Geometry: see drawing. Coordinates: mm, zero at the bounding-box minimum. A direction names the side the tool comes from. Round coordinates to 2 decimals unless told otherwise and drop trailing zeros. Order: outer loops, then holes, each group sorted by start corner. A loop starts at its lowest first (then second) coordinate and runs counter-clockwise, first axis right, second up. Notation, with made-up numbers: (40, -0.5) -> (86, -0.5) arc R28 cw to (86, 32.5) -> close; hole circle Ø8 at (87.25, 86.25). An arc over 180 degrees is marked (long way). Answer as CSV lines item,"result". Start each with the question number.
(1) Section query A-A (x = 36). Output: boundary loops of the cut face in (y, z).
(2) Line query: line 1 along X through (y, z) = (3.8, 60.29); line 2 along X through (y, z) = (0.3, 5); line 3 along X through (y, z) = (3.5, 39.5). Output: solid intervals per line, ascending. Write a range as from..to.
(3) Contact query for flat-ended pins moving along their axis: P1, Ø0.9, axis at y = 1, z = 49.5, coming from the +X side; P2, Ø12, axis at x = 13.5, z = 42, coming from the -Y side; P3, Ø2.5, axis at y = 2, z = 37, coming from the -X side; P4, Ø1, axis at x = 16.5, z = 56.5, coming from the -Y side. Output: stop coordinate, or through.
(4) Section query C-C (y = 3.9). Output: boundary loops of the cut face in (x, z).
(5) Section query D-D (x = 23). Output: boundary loops of the cut face in (y, z), plus the area to 3 significant figures.
(6) Section query B-B (z = 5.5). Output: boundary loops of the cut face in (x, y).
(7) Set-up query: the marked faces 1, 2 and 3. Return all of +Z, -Z, +X, -X, +Y, -Y with unobstructed straight access to the full face (end or side cutting, diameter ignored); none if empty.
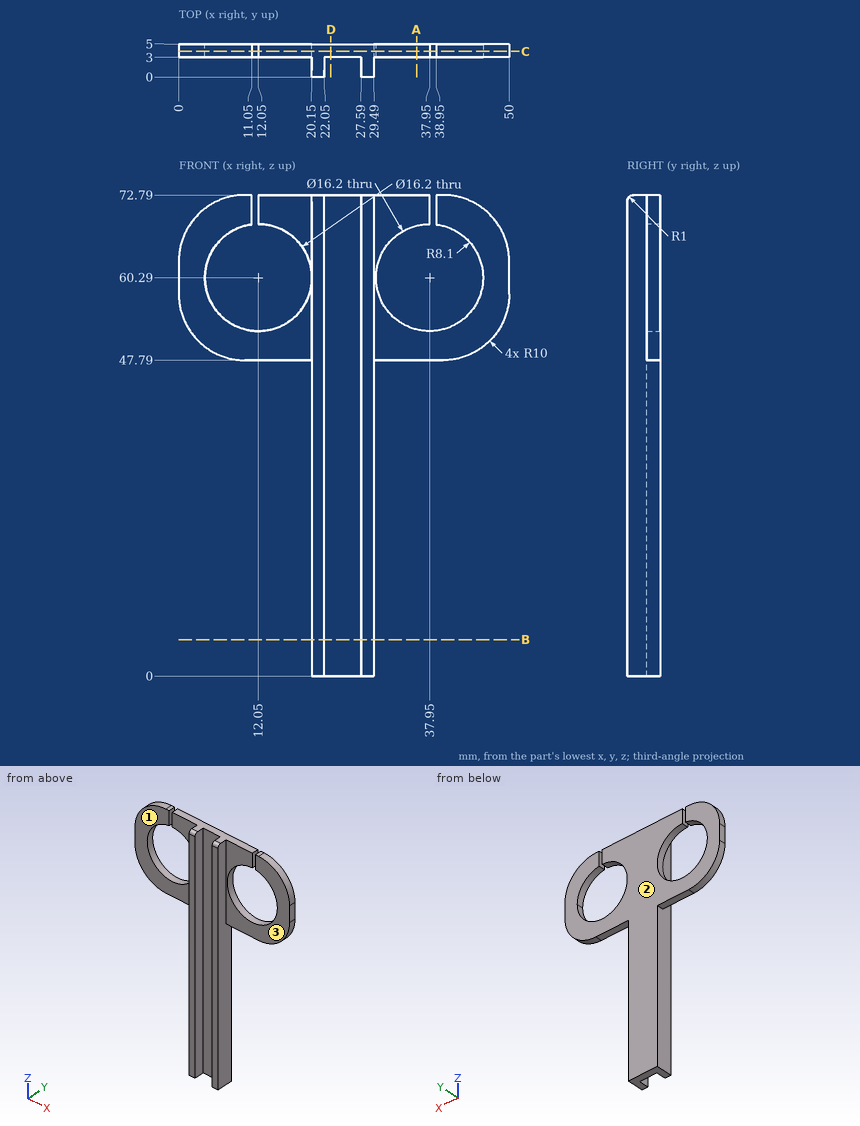
Answer block:
1,outline,"(3, 47.79) -> (5, 47.79) -> (5, 52.43) -> (3, 52.43) -> close; (3, 68.15) -> (5, 68.15) -> (5, 72.79) -> (3, 72.79) -> close"
2,line 1,"0..3.95, 20.15..29.85, 46.05..50"
2,line 2,"20.15..22.05, 27.59..29.49"
2,line 3,"20.15..29.49"
3,P1,"x = 29.49"
3,P2,"y = 3"
3,P3,"x = 20.15"
3,P4,"through"
4,outline,"(0, 57.79) arc R10 ccw to (10, 47.79) -> (20.15, 47.79) -> (20.15, 0) -> (29.49, 0) -> (29.49, 47.79) -> (40, 47.79) arc R10 ccw to (50, 57.79) -> (50, 62.79) arc R10 ccw to (40, 72.79) -> (38.95, 72.79) -> (38.95, 68.33) arc R8.1 cw (long way) to (37.95, 68.39) -> (37.95, 72.79) -> (12.05, 72.79) -> (12.05, 68.39) arc R8.1 cw (long way) to (11.05, 68.33) -> (11.05, 72.79) -> (10, 72.79) arc R10 ccw to (0, 62.79) -> close"
5,outline,"(3, 0) -> (5, 0) -> (5, 72.79) -> (3, 72.79) -> close"
5,area,"146 mm2"
6,outline,"(20.15, 0) -> (22.05, 0) -> (22.05, 3) -> (27.59, 3) -> (27.59, 0) -> (29.49, 0) -> (29.49, 5) -> (20.15, 5) -> close"
7,face 1,"+Z, -Z, -X, -Y"
7,face 2,"+Z, -Z, +X, -X, +Y"
7,face 3,"+Z, -Z, +X, -Y"
